Can you work these out from the model? Positions are in its coordinate system, mm. A direction names the side the tool comes from. Round coordinates to 2 decimals unless told otherwise and drop trailing zeros. Order: outer loops, then holes, each group sorted by start corner. A loop starts at its lowest first (then second) coordinate and runs counter-clockwise, first axis right, second up. Notation, with made-up numbers: M 89.25,-27.5 L 141.25,-27.5 A26 cw 141.25,-8.5 Z; hole C 61,59.5 d3. An arc over 180 degrees is marked long. Answer as CSV lines item,"result". Start each with the question number.
from build123d import *

# Parameters (mm, degrees)
BOSS_EXTRUDE1_DEPTH = 100
SKETCH2_R           = 70
CUT_EXTRUDE1_DEPTH  = 100
SKETCH3_R           = 70
BOSS_EXTRUDE2_DEPTH = 100


with BuildPart() as part:
    # Sketch1 → Boss-Extrude1 (new body)
    with BuildSketch(Plane(origin=(0, 0, 0), x_dir=(1, 0, 0), z_dir=(0, 1, 0))):
        with BuildLine():
            Line((-242.625717576, 275.741810419), (-242.625717576, 275.992438563))
            Line((-242.625717576, 275.992438563), (157.374282424, 275.992438563))
            Line((157.374282424, 275.992438563), (157.374282424, 275.741810419))
            ThreePointArc((157.374282424, 275.741810419), (322.374282424, 225.992438563), (157.374282424, 176.243066708))
            Line((157.374282424, 176.243066708), (157.374282424, 175.992438563))
            Line((157.374282424, 175.992438563), (-242.625717576, 175.992438563))
            Line((-242.625717576, 175.992438563), (-242.625717576, 176.243066708))
            ThreePointArc((-242.625717576, 176.243066708), (-407.625717576, 225.992438563), (-242.625717576, 275.741810419))
        make_face()
    extrude(amount=BOSS_EXTRUDE1_DEPTH)

    # Sketch2 → Cut-Extrude1 (cut)
    with BuildSketch(Plane(origin=(0, 100, 0), x_dir=(1, 0, 0), z_dir=(0, 1, 0))):
        with Locations(Location((-317.625717576, 225.992438563, 0), (0, 0, 270))):
            Circle(SKETCH2_R)
    extrude(amount=-CUT_EXTRUDE1_DEPTH, mode=Mode.SUBTRACT)

    # Sketch3 → Boss-Extrude2 (add)
    with BuildSketch(Plane(origin=(0, 100, 0), x_dir=(1, 0, 0), z_dir=(0, 1, 0))):
        with Locations(Location((232.374282424, 225.992438563, 0), (0, 0, 270))):
            Circle(SKETCH3_R)
    extrude(amount=BOSS_EXTRUDE2_DEPTH)


solid = part.part
(1) I want a section at D-D on x = -333. Write out the boundary of the cut face in (y, z).
(2) I want a section at A-A on z = -209.5. Write out the boundary of the cut face in (x, y).
(3) For faces 1 (the flat face through (-40, 49, -175.992)), 2 (the cylindrical face through (322.317, 49.3, -229.212)), 3 (the flat face through (-45, 49, -275.992)), which set-ups out of +Z, -Z, +X, -X, +Y, -Y let a thin tool reach every point of the face, with its end or its side?
(4) I'm going to push flat-ended pins straight in: P1, Ø6, axis at y = 80, z = -178.5, coming from the -X side; P2, Ø1.5, axis at y = 49, z = -262, coming from the +X side; P3, Ø2, axis at x = 94.5, y = 74.5, coming from the -Z side; P4, Ø8, axis at x = -179, z = -245.5, coming from the -Y side. Where does each tip first touch, or does it pass through?
(5) If we mould it in two halves opening along X, with no side actions, what happens to faces 4 (the flat face through (-38, 100, -227)), 5 (the cylindrical face through (-386, 51, -241)), 6 (the cylindrical face through (164, 149, -241))? For each: +X half, -X half, draft (parallel to the pull), parting line (faces both ways), or undercut.
(6) If I drill on line 1 along X through (y, z) = (29, -166.5); line 2 along Y through (x, z) = (-115, -219); line 3 along X through (y, z) = (66, -280.5), over which ranges is the centre line in solid material (lowest first)?
(7) I want a section at B-B on x = 278. Write out the boundary of the cut face in (y, z).
(8) I want a section at C-C on y = 53.5. Write out the boundary of the cut face in (x, z), and give its area (3 significant figures).
From the geometry:
1,outline,"M 0,-314.67 L 100,-314.67 L 100,-294.28 L 0,-294.28 Z; M 0,-157.7 L 100,-157.7 L 100,-137.32 L 0,-137.32 Z"
2,outline,"M -406.1,0 L -385.66,0 L -385.66,100 L -406.1,100 Z; M -249.6,0 L 320.85,0 L 320.85,100 L 300.4,100 L 300.4,200 L 164.34,200 L 164.34,100 L -249.6,100 Z"
3,face 1,"+Z, +Y, -Y"
3,face 2,"+Y, -Y"
3,face 3,"-Z, +Y, -Y"
4,P1,"x = -395.86"
4,P2,"x = 315.18"
4,P3,"z = -275.99"
4,P4,"y = 0"
5,face 4,"draft"
5,face 5,"undercut"
5,face 6,"parting line"
6,line 1,"-385.16 to -354.51, -280.74 to -250.09, 164.84 to 299.91"
6,line 2,"0 to 100"
6,line 3,"-389.24 to -361.55, -273.71 to -246.01, 160.76 to 303.99"
7,outline,"M 0,-303.57 L 100,-303.57 L 100,-279.08 L 200,-279.08 L 200,-172.9 L 100,-172.9 L 100,-148.41 L 0,-148.41 Z"
8,outline,"M -242.63,-275.99 L 157.37,-275.99 L 157.37,-275.74 A90 ccw long 157.37,-176.24 L 157.37,-175.99 L -242.63,-175.99 L -242.63,-176.24 A90 ccw long -242.63,-275.74 Z; hole C -317.63,-225.99 d140"
8,area,"73,500 mm²"
